Autodesk Inventor part; units mm, degrees
ref_plane "YZ Plane" through (0, 0, 0) normal (1, 0, 0) x (0, 1, 0)
ref_plane "XZ Plane" through (0, 0, 0) normal (0, 1, 0) x (-1, 0, 0)
ref_plane "XY Plane" through (0, 0, 0) normal (0, 0, 1) x (1, 0, 0)
sketch "Эскиз1" plane through (0, 0, 0) normal (0, 1, 0) x (-1, 0, 0)
  circle A0 centre (0, 0) radius 4.95
  circle A1 centre (0, 0) radius 5.95
  line L0 (0, 0) -> (4.748, 3.586)
  line L1 (0, 0) -> (4.748, -3.586)
  point P0 (3.95, -2.9833)
  point P1 (3.95, 2.9833)
  dimension "d0" = 9.9
  dimension "d1" = 11.9
extrude "Выдавливание1" add sketch "Эскиз1" along normal blind 30 contours A0 L1 A1 L0 picked at (4.1379, 3.7388)
sketch "Эскиз2" plane through (0, 30, 0) normal (0, 1, 0) x (1, 0, 0)
  arc A0 (-3.95, -2.9833) -> (-4.8427, -2.4534) centre (-6.6513, -6.5172) ccw
  arc A1 (-4.8427, -2.4534) -> (-5.9996, -4.2591) centre (-5.277, -3.4486) ccw
  line L0 (-5.9996, -4.2591) -> (-5.3283, -3.4047)
  arc A2 (-4.7494, -3.5714) -> (-5.3283, -3.4047) centre (-5.1177, -3.7619) ccw
  line L1 (-3.95, -2.9833) -> (-4.748, -3.586)
  line L2 (-4.748, -3.586) -> (-3.95, -2.9833)
  line L3 (-4.748, -3.586) -> (-4.7494, -3.5714)
  line L4 (-0.0151, 0) -> (-3.489, 0)
  arc A3 (-4.8427, 2.4534) -> (-3.95, 2.9833) centre (-6.6513, 6.5172) ccw
  arc A4 (-5.3283, 3.4047) -> (-4.7494, 3.5714) centre (-5.1177, 3.7619) ccw
  line L5 (-3.95, 2.9833) -> (-4.748, 3.586)
  line L6 (-4.748, 3.586) -> (-3.95, 2.9833)
  line L7 (-4.748, 3.586) -> (-4.7494, 3.5714)
  arc A5 (-5.9996, 4.2591) -> (-4.8427, 2.4534) centre (-5.277, 3.4486) ccw
  line L8 (-5.9996, 4.2591) -> (-5.3283, 3.4047)
  point P0 (-3.95, 2.9833)
  point P1 (-4.748, -3.586)
  point P2 (-5.3694, -4.0591)
  point P3 (-4.748, 3.586)
  point P4 (-5.3694, 4.0591)
  point P5 (-4.748, 3.586)
  dimension "d25" = 1.0859
sketch "Эскиз3" plane through (0, 30, 0) normal (0, 1, 0) x (1, 0, 0)
  arc A0 (-4.748, -3.586) -> (-4.748, 3.586) centre (0, 0) ccw
  line L0 (11.5, -6.95) -> (11.5, 6.95)
  arc A1 (-3.95, -2.9833) -> (-3.95, 2.9833) centre (0, 0) ccw
  line L1 (0, -5.95) -> (0, -4.95)
  line L2 (0, 4.95) -> (0, 5.95)
  line L3 (11.5, 6.95) -> (11.5, 10.95)
  line L4 (11.5, -6.95) -> (11.5, -10.95)
  line L5 (0, 1.45) -> (0, 5.95)
  line L6 (11.5, -10.95) -> (0, -10.95)
  line L7 (0, -10.95) -> (0, -5.95)
  line L8 (11.5, 10.95) -> (0, 10.95)
  line L9 (0, 10.95) -> (0, 5.95)
  arc A2 (0, -4.95) -> (0, 4.95) centre (0, 0) ccw
  dimension "d13" = 4
  dimension "d14" = 4
  dimension "d22" = 21.9
  dimension "d23" = 6
extrude "Выдавливание3" add sketch "Эскиз3" against normal blind 30
ref_plane "РабПлоскость1" through (11.5, 20, 4.95) normal (1, 0, 0) x (0, 0, -1)
sketch "Эскиз4" plane through (11.5, 20, 4.95) normal (1, 0, 0) x (0, 0, -1)
  line L0 (4.95, -20) -> (4.95, 10)
  line L1 (1, 10) -> (8.9, 10)
  circle A0 centre (4.95, -12) radius 5
  line L2 (14.4, -20) -> (-4.5, -20)
  circle A1 centre (4.95, 2) radius 5
  line L3 (-4.5, 10) -> (14.4, 10)
  point P0 (7.3306, 10)
  point P1 (2.5694, 10)
  point P2 (4.95, 10)
  dimension "d15" = 10
  dimension "d16" = 8
  dimension "d17" = 10
  dimension "d18" = 8
extrude "Выдавливание4" cut sketch "Эскиз4" against normal blind 2
extrude "Выдавливание5" add sketch "Эскиз2" against normal blind 30
sketch "Эскиз5" plane through (0, 30, 0) normal (0, 1, 0) x (1, 0, 0)
  arc A0 (0, 5.95) -> (-4.748, 3.586) centre (0, 0) ccw
  line L0 (-4.748, 3.586) -> (-4.7494, 3.5714)
  arc A1 (-5.3283, 3.4047) -> (-4.7494, 3.5714) centre (-5.1177, 3.7619) ccw
  line L1 (-5.3283, 3.4047) -> (-5.9996, 4.2591)
  arc A2 (-5.9996, 4.2591) -> (-4.8427, 2.4534) centre (-5.277, 3.4486) ccw
  arc A3 (-4.8427, 2.4534) -> (-3.95, 2.9833) centre (-6.6513, 6.5172) ccw
  arc A4 (-3.95, -2.9833) -> (-3.95, 2.9833) centre (0, 0) ccw
  arc A5 (-3.95, -2.9833) -> (-4.8427, -2.4534) centre (-6.6513, -6.5172) ccw
  arc A6 (-4.8427, -2.4534) -> (-5.9996, -4.2591) centre (-5.277, -3.4486) ccw
  line L2 (-5.9996, -4.2591) -> (-5.3283, -3.4047)
  arc A7 (-4.7494, -3.5714) -> (-5.3283, -3.4047) centre (-5.1177, -3.7619) ccw
  line L3 (-4.7494, -3.5714) -> (-4.748, -3.586)
  arc A8 (-4.748, -3.586) -> (0, -5.95) centre (0, 0) ccw
  line L4 (0, -5.95) -> (0, -10.95)
  line L5 (0, -10.95) -> (11.5, -10.95)
  line L6 (11.5, -10.95) -> (11.5, 10.95)
  line L7 (11.5, 10.95) -> (0, 10.95)
  line L8 (0, 10.95) -> (0, 5.95)
  line L9 (0, 4.95) -> (0, 5.95)
  line L10 (0, -4.95) -> (0, -5.95)
extrude "Выдавливание6" [suppressed]
sketch "Эскиз6" plane through (11.5, 30, 10.95) normal (1, 0, 0) x (0, 0, -1)
  arc A0 (15.95, -22) -> (15.95, -22) centre (10.95, -22) ccw
  arc A1 (15.95, -8) -> (15.95, -8) centre (10.95, -8) ccw
  point P0 (10.95, -30)
extrude "Выдавливание7" [suppressed]
sketch "Эскиз7" plane through (11.5, 30, 10.95) normal (1, 0, 0) x (0, 0, -1)
  circle A0 centre (10.95, -8) radius 5
  circle A1 centre (10.95, -22) radius 5
  line L0 (0, 0) -> (21.9, 0)
  line L1 (0, 0) -> (0, -30)
  line L2 (21.9, -30) -> (0, -30)
  line L3 (21.9, 0) -> (21.9, -30)
  point P0 (10.95, -30)
properties part number "крепление маркера 10мм"
Build history of the part. All positions in model axes, mm. A direction names the side the tool comes from. Round coordinates to 2 decimals unless told otherwise and drop trailing zeros. Loops run counter-clockwise (first coordinate to the right, second up) from the corner with the lowest first, then second, coordinate; pieces in that order, holes last. Notation, with made-up numbers: (-18.5, -39.5) -> (3.5, -39.5) arc R6 cw to (3.5, -33.5) -> close; hole circle Ø1 at (56.25, 18.25). An arc over 180 degrees is marked (long way). One line per item, written item: value. Start each with the question number.
Q1. Cut at D-D on z = -8. List the corners of the cut face in (x, y).
Q2. Drop flat-ended pins along their axis: pin 1 Ø4 at (y, z) = (20, 7.5) entering from -X; pin 2 Ø9 at (y, z) = (22, 0) entering from +X; pin 3 Ø5.5 at (y, z) = (14, -7.5) entering from -X. Give the stop position or say it passes through.
Q3. Cut at A-A on z = 0. List the corners of the cut face in (x, y), plus the area to 4 significant figures.
Q4. 3-axis set-ups, long thin cutter, end or side, ignore diameter. For faces 1 (the face through (9.5, 8, 0)), 2 (the face through (0, 15, 8)), 3 (the face through (0, 15, -8)): which of +Z, -Z, +X, -X, +Y, -Y reach the whole face in a straight line?
Q5. Two-plate mould, pull along Z, no slides. Class faces 4 (the face through (9.5, 22, 0)), 5 (the face through (7, 30, 0)), 6 (the face through (-2.7, 14.8, -5.3)): released by +Z, released by -Z, zero draft, split by the parting line, or undercut.
Q6. Probe line 1 along Y through (x, z) = (10.55, 0); line 2 along Z through (x, y) = (9.9, 22); line 3 along X through (y, z) = (26, -7.25). List the from-to ranges inside material, lowest first.
Computed:
1. outline: (0, 0) -> (11.5, 0) -> (11.5, 30) -> (0, 30) -> close
2. pin 1: x = -2.27
2. pin 2: x = 9.5
2. pin 3: x = -3.58
3. outline: (4.95, 0) -> (11.5, 0) -> (11.5, 3) -> (9.5, 3) -> (9.5, 13) -> (11.5, 13) -> (11.5, 17) -> (9.5, 17) -> (9.5, 27) -> (11.5, 27) -> (11.5, 30) -> (4.95, 30) -> close
3. area: 156.5 mm²
4. face 1: +X
4. face 2: +Z, -X, +Y, -Y
4. face 3: -Z, -X, +Y, -Y
5. face 4: undercut
5. face 5: zero draft
5. face 6: released by -Z
6. line 1: 0 to 3, 13 to 17, 27 to 30
6. line 2: -10.95 to -5, 5 to 10.95
6. line 3: 0 to 11.5
